Part print with two shaded views. Sizes in mm from the minimum x, y, z corner. A direction names the side the tool comes from. Give positions to 0.01 mm unless a question says otherwise; leave off trailing zeros. Order: outer loops, then holes, each group sorted by start corner. A loop starts at its lowest first (then second) coordinate and runs counter-clockwise, first axis right, second up. Notation, with made-up numbers: M 19,-8.5 L 31,-8.5 A20 cw 31,-4.5 Z; hole C 6.25,-11 d8. An arc over 180 degrees is marked long. Answer as CSV lines item,"result".
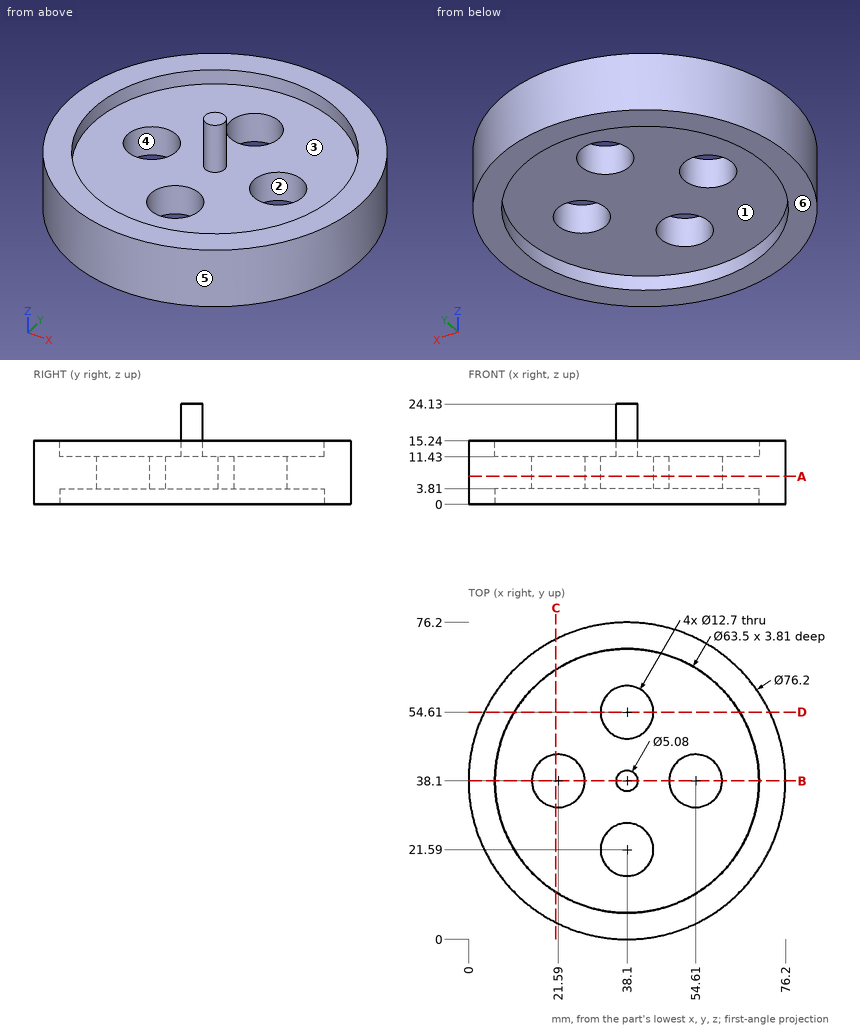
Item 1: Probe line 1 along Y through (x, z) = (38.1, 12.45); line 2 along Y through (x, z) = (38.1, 7.75); line 3 along Y through (x, z) = (38.1, 2.25). List the from-to ranges inside material, lowest first. Write a range as from..to.
Geometry says:
line 1,"y = 0..6.35, 35.56..40.64, 69.85..76.2"
line 2,"y = 0..15.24, 27.94..48.26, 60.96..76.2"
line 3,"y = 0..6.35, 69.85..76.2"
Item 2: 3-axis set-ups, long thin cutter, end or side, ignore diameter. For the marked faces 1, 2 and 3: which of +Z, -Z, +X, -X, +Y, -Y reach the whole face in a straight line?
Geometry says:
face 1,"-Z"
face 2,"+Z, -Z"
face 3,"+Z"
Item 3: Band-saw the part on A-A (z = 6.75). Give the cut face in (x, y), and give its area (3 significant figures).
Geometry says:
outline,"C 38.1,38.1 d76.2; hole C 21.59,38.1 d12.7; hole C 38.1,21.59 d12.7; hole C 38.1,54.61 d12.7; hole C 54.61,38.1 d12.7"
area,"4,050 mm2"
Item 4: Drop flat-ended pins along their axis: pin 1 (4 mm diameter, centred on x = 46, z = 8, fed in from -Y); pin 2 (8 mm diameter, centred on x = 48, y = 48.5, fed in from -Z); pin 3 (6 mm diameter, centred on y = 10, z = 5, fed in from -X); pin 4 (10 mm diameter, centred on x = 38.1, y = 54.61, fed in from +Z). Give the stop position or say it passes through.
Geometry says:
pin 1,"stops at y = 0.46"
pin 2,"stops at z = 3.81"
pin 3,"stops at x = 9.44"
pin 4,"passes through"
Item 5: Band-saw the part on B-B (y = 38.1). Give the cut face in (x, z), and give its area (3 significant figures).
Geometry says:
outline,"M 0,0 L 6.35,0 L 6.35,3.81 L 15.24,3.81 L 15.24,11.43 L 6.35,11.43 L 6.35,15.24 L 0,15.24 Z; M 27.94,3.81 L 48.26,3.81 L 48.26,11.43 L 40.64,11.43 L 40.64,24.13 L 35.56,24.13 L 35.56,11.43 L 27.94,11.43 Z; M 60.96,3.81 L 69.85,3.81 L 69.85,0 L 76.2,0 L 76.2,15.24 L 69.85,15.24 L 69.85,11.43 L 60.96,11.43 Z"
area,"548 mm2"
Item 6: Band-saw the part on D-D (y = 54.61). Give the cut face in (x, z), and give its area (3 significant figures).
Geometry says:
outline,"M 3.76,0 L 10.98,0 L 10.98,3.81 L 31.75,3.81 L 31.75,11.43 L 10.98,11.43 L 10.98,15.24 L 3.76,15.24 Z; M 44.45,3.81 L 65.22,3.81 L 65.22,0 L 72.44,0 L 72.44,15.24 L 65.22,15.24 L 65.22,11.43 L 44.45,11.43 Z"
area,"537 mm2"
Item 7: Band-saw the part on C-C (x = 21). Give the cut face in (y, z), and give its area (3 significant figures).
Geometry says:
outline,"M 4.05,0 L 11.35,0 L 11.35,3.81 L 31.78,3.81 L 31.78,11.43 L 11.35,11.43 L 11.35,15.24 L 4.05,15.24 Z; M 44.42,3.81 L 64.85,3.81 L 64.85,0 L 72.15,0 L 72.15,15.24 L 64.85,15.24 L 64.85,11.43 L 44.42,11.43 Z"
area,"534 mm2"
Item 8: Pull direction X, two halves, no side cores. Call the marked faces 4, 5 and 6: released by +X, released by -X, zero draft, split by the parting line, or undercut.
Geometry says:
face 4,"undercut"
face 5,"split by the parting line"
face 6,"zero draft"
